Input: dimensioned drawing with shaded views. Units: mm. Origin: part minimum x, y, z. Give positions to 0.01 mm unless a question says otherwise; leave off trailing zeros. Write each loop counter-clockwise with the first axis right and the second up, starting at its lowest first coordinate (ties: lowest second). Pieces come first, ordered by that corner, then holes. Notation, with made-up numbers: (35.25, 7) -> (43.25, 7) arc R18 ccw to (43.25, 11) -> close; hole circle Ø3 at (59.5, -25.75). An arc over 180 degrees is marked (long way). Return JSON: item names as keys, results as strings. Group by question number.
Item 1: Mould query, pull axis X, two halves, no side actions, for the marked faces 1, 2 and 3. Classes: released by +X, released by -X, zero draft, split by the parting line, or undercut.
Item 2: Line query: line 1 (Y direction, x = 9.8, z = 79.5); line 2 (X direction, y = 9.5, z = 18); line 3 (Z direction, x = 9.5, y = 4). Output: solid intervals per line, ascending. Write a range as [from, to].
Item 3: Section A-A, the plane x = 9.8. Return loops of the section in (y, z), then the cut area to 3 significant figures.
Item 4: Pin query (flat end, axial travel): P1, Ø5, axis at x = 7, z = 29.5, coming from the +Y side; P2, Ø6, axis at x = 3, z = 77, coming from the -Y side; P3, Ø3, axis at y = 15, z = 58, coming from the -X side. Return the tip coordinate at first contact, or that it passes through.
Item 5: Section C-C, the plane z = 83. Return loops of the section in (x, y).
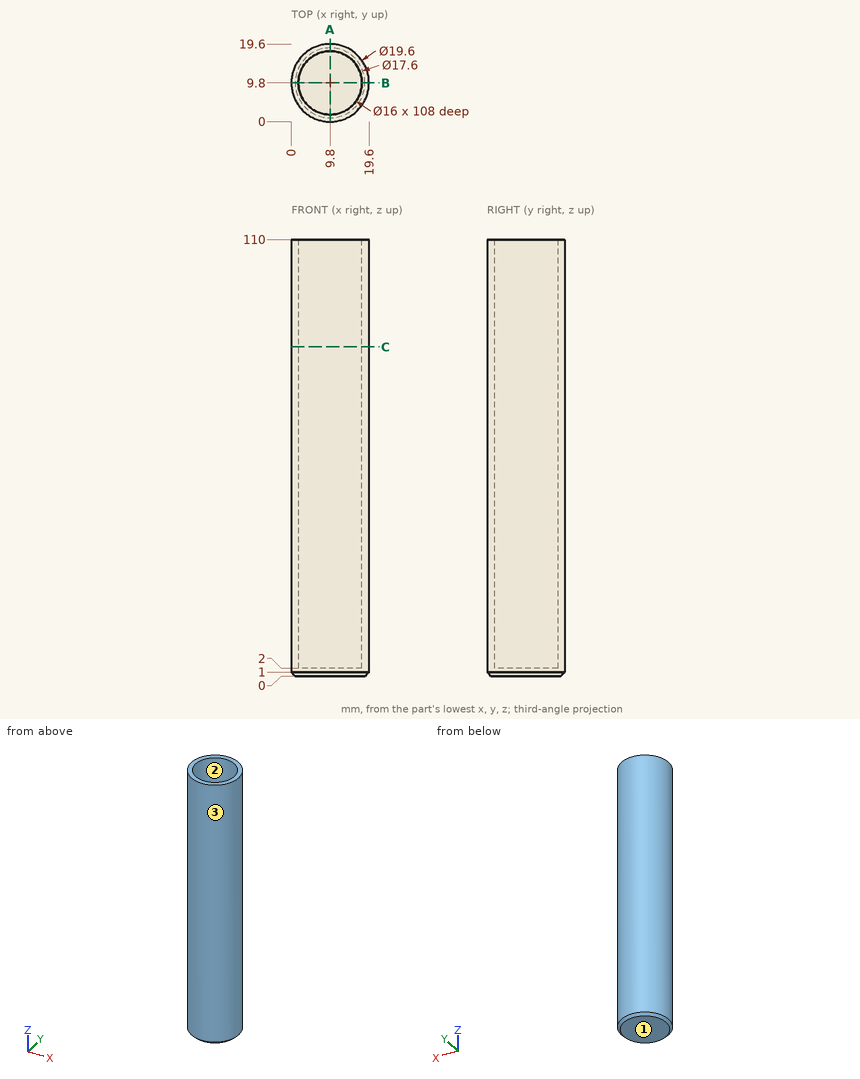
Answer below:
{
 "1": {"face 1": "zero draft", "face 2": "undercut", "face 3": "split by the parting line"},
 "2": {"line 1": "y = [0, 1.8], [17.8, 19.6]", "line 2": "x = [0, 1.81], [17.79, 19.6]", "line 3": "z = [0, 2]"},
 "3": {"outline": "(0, 1) -> (1, 0) -> (18.6, 0) -> (19.6, 1) -> (19.6, 110) -> (17.8, 110) -> (17.8, 2) -> (1.8, 2) -> (1.8, 110) -> (0, 110) -> close", "area": "427 mm2"},
 "4": {"P1": "stops at y = 19.6", "P2": "stops at y = 0.77", "P3": "stops at x = 0.73"},
 "5": {"outline": "circle Ø19.6 at (9.8, 9.8); hole circle Ø16 at (9.8, 9.8)"}
}
